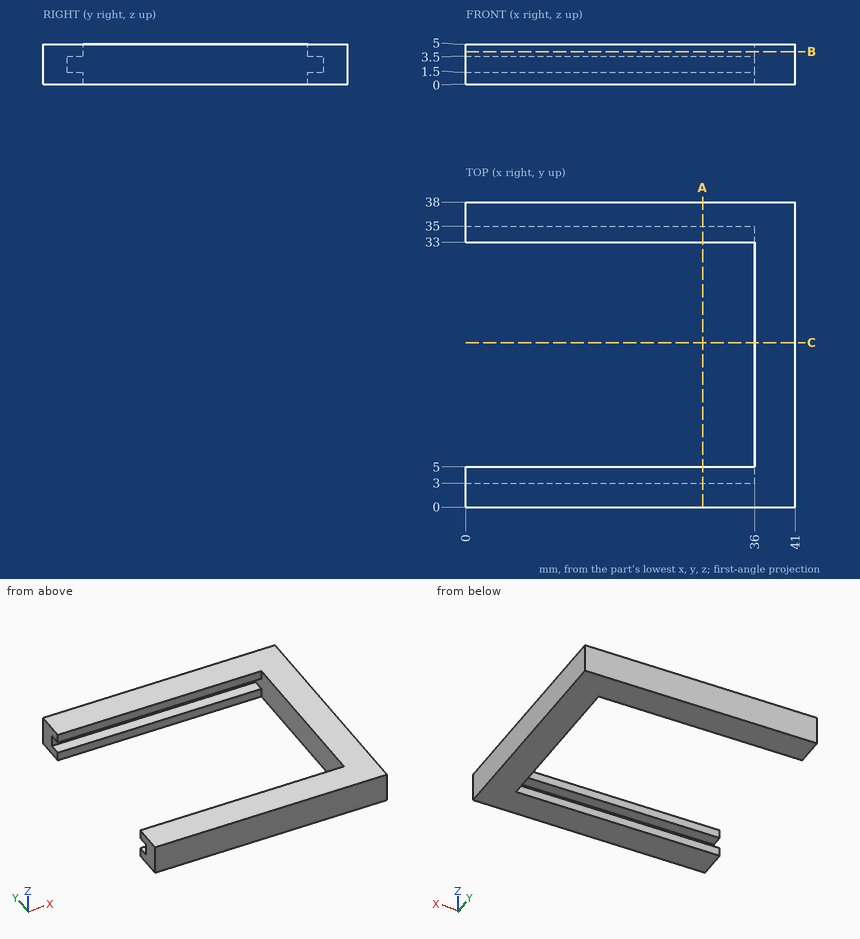
Could you check a few things on this drawing? It's one solid part, dimensions in mm from its lowest x, y, z. Round coordinates to 2 decimals unless told otherwise and drop trailing zeros. Write each loop counter-clockwise with the first axis right and the second up, starting at its lowest first coordinate (ties: lowest second). Pieces come first, ordered by that corner, then holes. Notation, with made-up numbers: (6.5, 46.5) -> (31.5, 46.5) arc R15 cw to (31.5, 50.5) -> close; hole circle Ø4 at (64, 86). An arc over 180 degrees is marked (long way). One line per question, with ' | ' between items. Start each with the question number.
1) Suppose I cut it at A-A on x = 29.5. Write out the boundary of the cut face in (y, z).
2) Suppose I cut it at B-B on z = 4.05. Write out the boundary of the cut face in (x, y), then the cut area to 3 significant figures.
3) I'm going to push a flat-ended pin straight in: P1, Ø12, axis at x = 32.5, y = 9.5, coming from the +Z side. Where does the tip first touch, or does it pass through?
4) I need wall thicknesses on line 1 (Y direction, x = 28, z = 1); line 2 (Y direction, x = 23, z = 2.25); line 3 (Z direction, x = 11, y = 3.5). Which ranges of each line are inside material? Lowest first, please. Write a range as [from, to].
5) Suppose I cut it at C-C on y = 20.5. Write out the boundary of the cut face in (x, z).
Return value:
1) outline: (0, 0) -> (5, 0) -> (5, 1.5) -> (3, 1.5) -> (3, 3.5) -> (5, 3.5) -> (5, 5) -> (0, 5) -> close; (33, 0) -> (38, 0) -> (38, 5) -> (33, 5) -> (33, 3.5) -> (35, 3.5) -> (35, 1.5) -> (33, 1.5) -> close
2) outline: (0, 0) -> (41, 0) -> (41, 38) -> (0, 38) -> (0, 33) -> (36, 33) -> (36, 5) -> (0, 5) -> close | area: 550 mm2
3) P1: stops at z = 5
4) line 1: y = [0, 5], [33, 38] | line 2: y = [0, 3], [35, 38] | line 3: z = [0, 1.5], [3.5, 5]
5) outline: (36, 0) -> (41, 0) -> (41, 5) -> (36, 5) -> close
